Work out the finished part from the listing and answer in its coordinate system (mm). Face numbers are marked on the shaded views. A direction names the side the tool comes from. Round coordinates to 2 decimals unless told otherwise and drop trailing zeros. Loops run counter-clockwise (first coordinate to the right, second up) from the corner with the lowest first, then second, coordinate; pieces in that order, holes last.
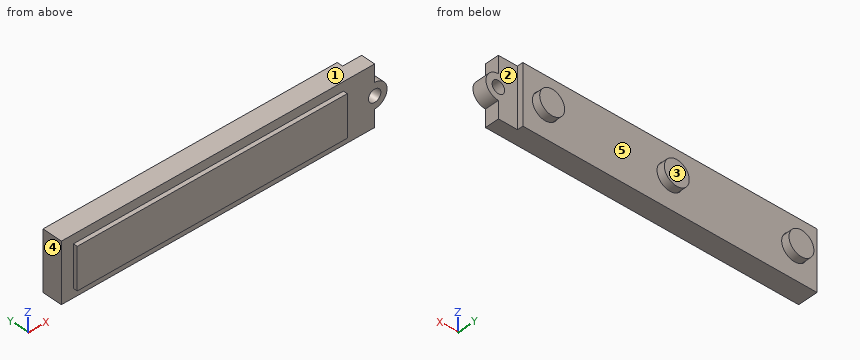
```python
from build123d import *

# Parameters (mm, degrees)
SKETCH1_W           = 99.568
SKETCH1_H           = 18.1102
BOSS_EXTRUDE1_DEPTH = 6.096
SKETCH2_W           = 9.652
SKETCH2_H           = 18.1102
CUT_EXTRUDE1_DEPTH  = 1.778
SKETCH3_R           = 1.905
CUT_EXTRUDE2_DEPTH  = 5.318
SKETCH4_R           = 3.937
CUT_EXTRUDE3_DEPTH  = 1.27
SKETCH5_W           = 82.55
SKETCH5_H           = 12.7
BOSS_EXTRUDE2_DEPTH = 1.27
CUT_EXTRUDE4_DEPTH  = 6.588
SKETCH8_R           = 3.81
BOSS_EXTRUDE3_DEPTH = 3.556


with BuildPart() as part:
    # Sketch1 → Boss-Extrude1 (new body)
    with BuildSketch(Plane(origin=(0, 0, 0), x_dir=(1, 0, 0), z_dir=(0, 1, 0))):
        with Locations((-66.378666667, 25.894273737)):
            Rectangle(SKETCH1_W, SKETCH1_H)
    extrude(amount=BOSS_EXTRUDE1_DEPTH)

    # Sketch2 → Cut-Extrude1 (cut)
    with BuildSketch(Plane(origin=(0, 6.096, 0), x_dir=(1, 0, 0), z_dir=(0, 1, 0))):
        with Locations((-21.420666667, 25.894273737)):
            Rectangle(SKETCH2_W, SKETCH2_H)
    extrude(amount=-CUT_EXTRUDE1_DEPTH, mode=Mode.SUBTRACT)

    # Sketch3 → Cut-Extrude2 (cut, through all)
    with BuildSketch(Plane(origin=(0, 4.318, 0), x_dir=(1, 0, 0), z_dir=(0, 1, 0))):
        with Locations((-20.404666667, 25.894273737)):
            Circle(SKETCH3_R)
    extrude(amount=-CUT_EXTRUDE2_DEPTH, mode=Mode.SUBTRACT)

    # Sketch4 → Cut-Extrude3 (cut)
    with BuildSketch(Plane(origin=(0, 6.096, 0), x_dir=(1, 0, 0), z_dir=(0, 1, 0))):
        with Locations((-33.104666667, 25.894273737)):
            Circle(SKETCH4_R)
        with Locations((-71.204666667, 25.894273737)):
            Circle(SKETCH4_R)
        with Locations((-109.304666667, 25.894273737)):
            Circle(SKETCH4_R)
    extrude(amount=-CUT_EXTRUDE3_DEPTH, mode=Mode.SUBTRACT)

    # Sketch5 → Boss-Extrude2 (add)
    with BuildSketch(Plane.XZ):
        with Locations((-71.204666667, -25.894273737)):
            Rectangle(SKETCH5_W, SKETCH5_H)
    extrude(amount=BOSS_EXTRUDE2_DEPTH)

    # Sketch7 → Cut-Extrude4 (cut, through all)
    with BuildSketch(Plane(origin=(0, 4.318, 0), x_dir=(1, 0, 0), z_dir=(0, 1, 0))):
        with BuildLine():
            Line((-16.594666667, 34.949373737), (-20.404666667, 34.949373737))
            Line((-20.404666667, 34.949373737), (-20.404666667, 29.680045052))
            ThreePointArc((-20.404666667, 29.680045052), (-16.618895352, 25.894273737), (-20.404666667, 22.108502422))
            Line((-20.404666667, 22.108502422), (-20.404666667, 16.839173737))
            Line((-20.404666667, 16.839173737), (-16.594666667, 16.839173737))
            Line((-16.594666667, 16.839173737), (-16.594666667, 34.949373737))
        make_face()
    extrude(amount=-CUT_EXTRUDE4_DEPTH, mode=Mode.SUBTRACT)

    # Sketch8 → Boss-Extrude3 (add)
    with BuildSketch(Plane(origin=(0, 4.826, 0), x_dir=(1, 0, 0), z_dir=(0, 1, 0))):
        with Locations((-33.104666667, 25.894273737)):
            Circle(SKETCH8_R)
        with Locations((-71.204666667, 25.894273737)):
            Circle(SKETCH8_R)
        with Locations((-109.304666667, 25.894273737)):
            Circle(SKETCH8_R)
    extrude(amount=BOSS_EXTRUDE3_DEPTH)


solid = part.part
```
1. Find section A-A (x = -48.5). Write down the section's boundary in (y, z), then the cut area to 3 significant figures.
Answer key:
outline: (-1.27, -32.24) - (0, -32.24) - (0, -34.95) - (6.1, -34.95) - (6.1, -16.84) - (0, -16.84) - (0, -19.54) - (-1.27, -19.54) - close
area: 127 mm2
2. Which of the six approach directions +Z, -Z, +X, -X, +Y, -Y give full straight-line access (tool end or side, diameter ignored) to the marked faces 1 and 2?
Answer key:
face 1: +Z, +X, -X, +Y, -Y
face 2: +Z, -Z, +X, +Y
3. Consider probe 1 along X at (y, z) = (7.25, -26); probe 2 along X at (y, z) = (4, -18.5); probe 3 along Y at (x, z) = (-86.5, -19.75). Determine where each line is inside the solid, lowest interval first.
Answer key:
probe 1: x = -113.11 to -105.5, -75.01 to -67.4, -36.91 to -29.3
probe 2: x = -116.16 to -20.4
probe 3: y = -1.27 to 6.1
4. Given pin 1 (1.4 mm diameter, centred on x = -71.5, y = -1, fed in from -Z); pin 2 (0.6 mm diameter, centred on y = -1, z = -25, fed in from +X); pin 3 (3 mm diameter, centred on x = -20.4, z = -25.89, fed in from +Y); pin 4 (4.5 mm diameter, centred on y = 1.5, z = -18.5, fed in from +X), each flat-ended and moving along its own axis, determine where each tip first touches the part or whether it passes through.
Answer key:
pin 1: stops at z = -32.24
pin 2: stops at x = -29.93
pin 3: passes through
pin 4: stops at x = -20.4
5. Find section B-B (y = 7). Write down the section's boundary in (x, z), then the cut area to 3 significant figures.
Answer key:
outline: circle Ø7.62 at (-109.3, -25.89); circle Ø7.62 at (-71.2, -25.89); circle Ø7.62 at (-33.1, -25.89)
area: 137 mm2
6. Determine the mould class of the marked faces 3, 4 and 5 for opening direction X: +X half, -X half, draft (parallel to the pull), parting line (faces both ways), or undercut.
Answer key:
face 3: draft
face 4: -X half
face 5: undercut
7. Find section C-C (y = 1.5). Write down the section's boundary in (x, z) (1 decimal).
Answer key:
outline: (-116.2, -34.9) - (-20.4, -34.9) - (-20.4, -29.7) arc R3.8 ccw to (-20.4, -22.1) - (-20.4, -16.8) - (-116.2, -16.8) - close; hole circle Ø3.8 at (-20.4, -25.9)
